from build123d import *

# Parameters (mm, degrees)
SKETCH_1_R          = 0.75
SKETCH_1_W          = 13
SKETCH_1_H          = 23
SKETCH_1_R_2        = 1.5
EXTRUDE_1_DEPTH     = 1.5
SKETCH_2_W          = 6
SKETCH_2_H          = 1
CUT_EXTRUDE_1_DEPTH = 3
FILLET_1_R          = 0.3


with BuildPart() as part:
    # 草图1 → 凸台-拉伸1 (new body, symmetric)
    with BuildSketch(Plane.XY):
        with BuildLine():
            ThreePointArc((-10, -8), (0, -18), (10, -8))
            Line((10, -8), (10, 6))
            Line((10, 6), (4.955472685, 43.54580062))
            ThreePointArc((4.955472685, 43.54580062), (-2.725773115, 47.071677579), (-2.618575221, 38.62053245))
            ThreePointArc((-2.618575221, 38.62053245), (-0.423906888, 35.714832413), (-0.782117822, 32.091112401))
            Line((-0.782117822, 32.091112401), (-10, 14))
            Line((-10, 14), (-10, -8))
        make_face()
        with Locations((0, -13.7)):
            Circle(SKETCH_1_R, mode=Mode.SUBTRACT)
        Rectangle(SKETCH_1_W, SKETCH_1_H, mode=Mode.SUBTRACT)
        with Locations((0, 13.7)):
            Circle(SKETCH_1_R, mode=Mode.SUBTRACT)
        with Locations((0, 42.88)):
            Circle(SKETCH_1_R_2, mode=Mode.SUBTRACT)
        Polygon((5.562298916, 16.5), (-5.359207663, 16.5), (3.283346167, 33.461966942), align=None, mode=Mode.SUBTRACT)
    extrude(amount=EXTRUDE_1_DEPTH, both=True)

    # 草图2 → 切除-拉伸1 (cut)
    with BuildSketch(Plane.XY.offset(1.5)):
        with Locations((0, -12)):
            Rectangle(SKETCH_2_W, SKETCH_2_H)
    extrude(amount=-CUT_EXTRUDE_1_DEPTH, mode=Mode.SUBTRACT)

    # 圆角1
    fillet_1_edges = [part.edges().sort_by_distance(p)[0] for p in [
        (-3, -11.5, 0),
        (3, -11.5, 0),
        (3, -12.5, 0),
        (-3, -12.5, 0),
    ]]
    fillet(fillet_1_edges, radius=FILLET_1_R)


solid = part.part
Can you work these out from the model? Positions are in its coordinate system, mm. A direction names the side the tool comes from. Give positions to 0.01 mm unless a question says otherwise; leave off trailing zeros. Write each loop counter-clockwise with the first axis right and the second up, starting at its lowest first coordinate (ties: lowest second). Pieces come first, ordered by that corner, then holes. Notation, with made-up numbers: M -30,78 L 28,78 A13 ccw 28,86 Z; hole C 63.25,-16.75 d1. An arc over 180 degrees is marked long. Answer in a Markdown table with one row per item. Add a question column.
Item 1: Imagine slicing it at D-D, the plane x = 8.5. Write out the boundary of the cut face in (y, z), plus the area to 3 significant figures.
Item 2: Imagine slicing it at C-C, the plane y = -13.7. Write out the boundary of the cut face in (x, z).
Item 3: On a 3-axis mill with a long thin cutter (end or side, diameter ignored), from which of +Z, -Z, +X, -X, +Y, -Y can I reach the whole of each face in a straight line? I mean faces 1 (the flat face through (0, 16.5, 0)), 2 (the flat face through (0, 15, -1.5)), 3 (the flat face through (-5.327, 23.172, 0.021)). Say none if no direction works.
Item 4: Imagine slicing it at A-A, the plane z = -0.4. Write out the boundary of the cut face in (x, y), plus the area to 3 significant figures.
Item 5: We'd pull the mould along Y, two halves only. Please class faces 4 (the flat face through (-10, 3, 0)), 5 (the flat face through (0, -12.5, 0)), 6 (the cylindrical face through (0, -18, 0)): released by +Y, released by -Y, zero draft, split by the parting line, or undercut.
Item 6: Please list where these lines run through material, in increasing order: L1, parallel to X at y = 3.5, z = 1.15; L2, parallel to Y at x = 1, z = 0.4; L3, parallel to Y at x = 0, z = -0.2.
Item 7: Imagine slicing it at B-B, the plane y = 28. Write out the boundary of the cut face in (x, z), plus the area to 3 significant figures.
Item 8: For pin 1 Ø1.5 at (x, z) = (4.5, 0.5) entering from +Y; pin 2 Ø1 at (x, z) = (-4, 0) entering from +Y; pin 3 Ø1 at (x, z) = (-3.5, -1) entering from +Y, each with a flat end and sliding along its axis, tell me the tip position at first contact or that it passes through.
Evaluation:
| question | item | result |
|---|---|---|
| 1 | outline | M -13.27,-1.5 L 17.16,-1.5 L 17.16,1.5 L -13.27,1.5 Z |
| 1 | area | 91.3 mm² |
| 2 | outline | M -8.22,-1.5 L -0.75,-1.5 L -0.75,1.5 L -8.22,1.5 Z; M 0.75,-1.5 L 8.22,-1.5 L 8.22,1.5 L 0.75,1.5 Z |
| 3 | face 1 | +Z, -Z |
| 3 | face 2 | -Z, +X, -X, +Y, -Y |
| 3 | face 3 | +Z, -Z, -X |
| 4 | outline | M -10,-8 A10 ccw 10,-8 L 10,6 L 4.96,43.55 A5 ccw long -2.62,38.62 A5 cw -0.78,32.09 L -10,14 Z; hole M -6.5,-11.5 L -3.3,-11.5 A0.3 cw -3,-11.8 L -3,-12.2 A0.3 ccw -2.7,-12.5 L 2.7,-12.5 A0.3 ccw 3,-12.2 L 3,-11.8 A0.3 cw 3.3,-11.5 L 6.5,-11.5 L 6.5,11.5 L -6.5,11.5 Z; hole M -5.36,16.5 L 5.56,16.5 L 3.28,33.46 Z; hole C 0,42.88 d3; hole C 0,-13.7 d1.5; hole C 0,13.7 d1.5 |
| 4 | area | 546 mm² |
| 5 | face 4 | zero draft |
| 5 | face 5 | undercut |
| 5 | face 6 | released by -Y |
| 6 | L1 | x = -10 to -6.5, 6.5 to 10 |
| 6 | L2 | y = -17.95 to -12.5, 11.5 to 16.5, 28.98 to 41.76, 44 to 47.78 |
| 6 | L3 | y = -18 to -14.45, -12.95 to -12.5, 11.5 to 12.95, 14.45 to 16.5, 27.02 to 41.38, 44.38 to 47.88 |
| 7 | outline | M -2.87,-1.5 L 0.5,-1.5 L 0.5,1.5 L -2.87,1.5 Z; M 4.02,-1.5 L 7.04,-1.5 L 7.04,1.5 L 4.02,1.5 Z |
| 7 | area | 19.2 mm² |
| 8 | pin 1 | stops at y = 46.19 |
| 8 | pin 2 | stops at y = 46.45 |
| 8 | pin 3 | stops at y = 46.88 |
